Read the model definition and answer for the solid it produces. Units are mm, in the model's axes. A direction names the side the tool comes from. Round coordinates to 2 decimals unless told otherwise and drop trailing zeros. Order: outer loops, then holes, each group sorted by start corner. A loop starts at its lowest first (then second) coordinate and runs counter-clockwise, first axis right, second up. Notation, with made-up numbers: (75.25, -28.75) -> (107.25, -28.75) arc R17 ccw to (107.25, -1.75) -> close; hole circle Ø4 at (-11, -7). An arc over 180 degrees is marked (long way). Use a Markdown table: item, result. Add a question column.
1. Section B-B, the plane y = -16 is taken. Give the vertices of the cut face in (x, z), then the cut area to 3 significant figures.
2. Section A-A, the plane x = -3 is taken. Give the vertices of the cut face in (y, z).
3. Given pin 1 (15 mm diameter, centred on x = 48, z = 26, fed in from -Y); pin 2 (4 mm diameter, centred on x = 62, z = 75.5, fed in from -Y); pin 3 (11 mm diameter, centred on x = 67.5, y = -25, fed in from +Z); pin 4 (4 mm diameter, centred on y = -36.5, z = -48.5, fed in from +X), each flat-ended and moving along its own axis, determine where each tip first touches the part or whether it passes through.
4. Consider L1, parallel to X at y = -21, z = 18.5; L2, parallel to X at y = -17.5, z = -17.5; L3, parallel to X at y = -32.5, z = -64. Determine where each line is inside the solid, lowest interval first. Write a range as [from, to].
5. Section C-C, the plane z = 2 is taken. Give the vertices of the cut face in (x, y).
6. For faces 4 (the face through (45, -5, 44)), 5 (the face through (25, -20, -56)), 6 (the face through (78, -10, 60)), determine the directions among +Z, -Z, +X, -X, +Y, -Y from which every point of the face is accessible in a straight line to the end or side of a thin tool.
7. Section D-D, the plane x = 48 is taken. Give the vertices of the cut face in (y, z), then the cut area to 4 significant figures.
8. The mould has two halves that part along Y. Classify faces 1 (the face through (13, -10, 60)), 2 (the face through (25, -17, 44)), 3 (the face through (-13.5, -12, 58)): +Y half, -Y half, draft (parallel to the pull), parting line (faces both ways), or undercut.
```python
from build123d import *

# Parameters (mm, degrees)
BOSS_EXTRUDE1_DEPTH = 115
BOSS_EXTRUDE2_DEPTH = 30
SKETCH3_W           = 55
SKETCH3_H           = 40
BOSS_EXTRUDE3_DEPTH = 10
SKETCH4_W           = 40
SKETCH4_H           = 40
BOSS_EXTRUDE4_DEPTH = 33
BOSS_EXTRUDE5_START = -5
BOSS_EXTRUDE5_DEPTH = 32
BOSS_EXTRUDE6_DEPTH = 115


with BuildPart() as part:
    # Sketch1 → Boss-Extrude1 (new body)
    with BuildSketch(Plane.XY):
        Polygon((0, 0), (90, 0), (90, -10), (65, -10), (65, -23), (60, -23), (60, -5), (30, -5), (30, -23), (25, -23), (25, -10), (0, -10), align=None)
    extrude(amount=BOSS_EXTRUDE1_DEPTH)

    # Sketch2 → Boss-Extrude2 (add)
    with BuildSketch(Plane(origin=(0, 0, 0), x_dir=(-1, 0, 0), z_dir=(0, 0, -1))):
        Polygon((-17.5, -10), (-17.5, 0), (-72.5, 0), (-72.5, -10), (-65, -10), (-65, -23), (-60, -23), (-60, -5), (-30, -5), (-30, -23), (-25, -23), (-25, -10), align=None)
    extrude(amount=BOSS_EXTRUDE2_DEPTH)

    # Sketch3 → Boss-Extrude3 (add)
    with BuildSketch(Plane(origin=(0, 0, -30), x_dir=(-1, 0, 0), z_dir=(0, 0, -1))):
        with Locations((-45, -20)):
            Rectangle(SKETCH3_W, SKETCH3_H)
    extrude(amount=BOSS_EXTRUDE3_DEPTH)

    # Sketch4 → Boss-Extrude4 (add)
    with BuildSketch(Plane(origin=(0, 0, -40), x_dir=(-1, 0, 0), z_dir=(0, 0, -1))):
        with Locations((-45, -20)):
            Rectangle(SKETCH4_W, SKETCH4_H)
    extrude(amount=BOSS_EXTRUDE4_DEPTH)

    # Sketch5 → Boss-Extrude5 (add)
    with BuildSketch(Plane.XZ.offset(40).offset(BOSS_EXTRUDE5_START)):
        Polygon((65, -73), (65, -40), (72.5, -40), (72.5, -30), (88, -30), (88, -73), align=None)
    extrude(amount=-BOSS_EXTRUDE5_DEPTH)

    # Sketch7 → Boss-Extrude6 (add)
    with BuildSketch(Plane.XY.offset(115)):
        Polygon((0, 0), (-15, 0), (-15, -23), (0, -23), (0, -21.5), (-13.5, -21.5), (-13.5, -1.5), (0, -1.5), align=None)
    extrude(amount=-BOSS_EXTRUDE6_DEPTH)


solid = part.part
```
Verdict:
| question | item | result |
|---|---|---|
| 1 | outline | (-15, 0) -> (-13.5, 0) -> (-13.5, 115) -> (-15, 115) -> close; (17.5, -40) -> (25, -40) -> (25, -73) -> (88, -73) -> (88, -30) -> (65, -30) -> (65, 115) -> (60, 115) -> (60, -30) -> (30, -30) -> (30, 115) -> (25, 115) -> (25, -30) -> (17.5, -30) -> close |
| 1 | area | 4,410 mm2 |
| 2 | outline | (-23, 0) -> (-21.5, 0) -> (-21.5, 115) -> (-23, 115) -> close; (-1.5, 0) -> (0, 0) -> (0, 115) -> (-1.5, 115) -> close |
| 3 | pin 1 | stops at y = -5 |
| 3 | pin 2 | stops at y = -23 |
| 3 | pin 3 | stops at z = 115 |
| 3 | pin 4 | stops at x = 88 |
| 4 | L1 | x = [-15, -13.5], [25, 30], [60, 65] |
| 4 | L2 | x = [25, 30], [60, 65] |
| 4 | L3 | x = [25, 88] |
| 5 | outline | (-15, -23) -> (0, -23) -> (0, -21.5) -> (-13.5, -21.5) -> (-13.5, -1.5) -> (0, -1.5) -> (0, -10) -> (25, -10) -> (25, -23) -> (30, -23) -> (30, -5) -> (60, -5) -> (60, -23) -> (65, -23) -> (65, -10) -> (90, -10) -> (90, 0) -> (-15, 0) -> close |
| 6 | face 4 | +Z, -Y |
| 6 | face 5 | -Z, -X, +Y, -Y |
| 6 | face 6 | +Z, +X, -Y |
| 7 | outline | (-40, -73) -> (0, -73) -> (0, 115) -> (-5, 115) -> (-5, -30) -> (-40, -30) -> close |
| 7 | area | 2,445 mm2 |
| 8 | face 1 | -Y half |
| 8 | face 2 | draft |
| 8 | face 3 | undercut |
